Read the model definition and answer for the solid it produces. Units are mm, in the model's axes. Face numbers are marked on the shaded views. Give positions to 0.01 mm unless a question says otherwise; leave off trailing zeros. Order: outer loops, then holes, each group sorted by start corner. A loop starts at its lowest first (then second) coordinate and runs counter-clockwise, first axis right, second up.
Item 1: The mould has two halves that part along Z. Classify the marked faces 1, 2 and 3: +Z half, -Z half, draft (parallel to the pull), parting line (faces both ways), or undercut.
Item 2: A cutting plane is placed at A-A (x = 11.75). Write down the section's boundary in (y, z), plus the area to 3 significant figures.
Item 3: A cutting plane is placed at B-B (y = 10). Write down the section's boundary in (x, z), plus the area to 3 significant figures.
Item 4: A cutting plane is placed at C-C (y = 35.5). Write down the section's boundary in (x, z).
Item 5: Find the intervals of material crossed by line 1 along Y through (x, z) = (11.75, 10.4); line 2 along X through (y, z) = (17, -30); line 3 along Z through (x, y) = (14.25, 46.5), in increasing order.
Item 6: A cutting plane is placed at D-D (z = -14). Write down the section's boundary in (x, y), plus the area to 3 significant figures.
Item 7: Given pin 1 Ø3 at (y, z) = (9, -11) entering from +X; pin 2 Ø12 at (y, z) = (7.5, -20.5) entering from -X; pin 3 Ø3.5 at (x, y) = (11.75, 10) entering from -Z; pin 4 Ø8 at (y, z) = (35, -21.5) entering from -X, each flat-ended and moving along its own axis, determine where each tip first touches the part or whether it passes through.
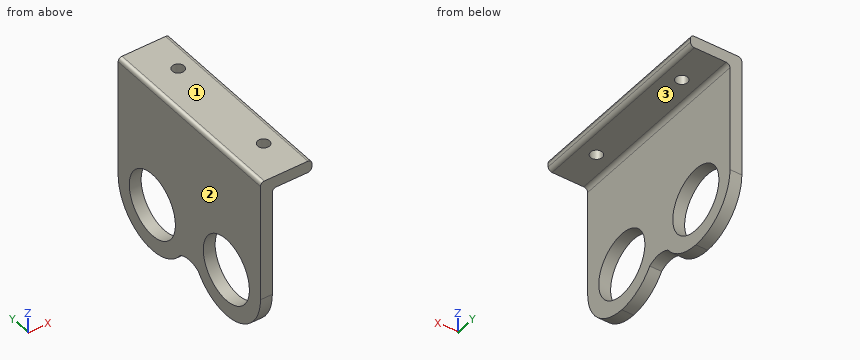
from build123d import *

# Parameters (mm, degrees)
BOSS_EXTRUDE1_DEPTH = 50
SKETCH2_R           = 1.5
CUT_EXTRUDE1_DEPTH  = 3
SKETCH3_R           = 8.1
CUT_EXTRUDE2_DEPTH  = 3


with BuildPart() as part:
    # Sketch1 → Boss-Extrude1 (new body)
    with BuildSketch(Plane(origin=(0, 0, 0), x_dir=(1, 0, 0), z_dir=(0, 1, 0))):
        with BuildLine():
            Line((3.75, 31.3125), (6.75, 31.3125))
            Line((6.75, 31.3125), (6.75, -7.6875))
            ThreePointArc((6.75, -7.6875), (7.042893219, -8.394606781), (7.75, -8.6875))
            Line((7.75, -8.6875), (15.75, -8.6875))
            ThreePointArc((15.75, -8.6875), (16.457106781, -8.980393219), (16.75, -9.6875))
            Line((16.75, -9.6875), (16.75, -10.6875))
            ThreePointArc((16.75, -10.6875), (16.457106781, -11.394606781), (15.75, -11.6875))
            Line((15.75, -11.6875), (4.75, -11.6875))
            ThreePointArc((4.75, -11.6875), (4.042893219, -11.394606781), (3.75, -10.6875))
            Line((3.75, -10.6875), (3.75, 31.3125))
        make_face()
    extrude(amount=BOSS_EXTRUDE1_DEPTH)

    # Sketch2 → Cut-Extrude1 (cut)
    with BuildSketch(Plane.XY.offset(11.6875)):
        with Locations((11.75, 40)):
            Circle(SKETCH2_R)
        with Locations((11.75, 10)):
            Circle(SKETCH2_R)
    extrude(amount=-CUT_EXTRUDE1_DEPTH, mode=Mode.SUBTRACT)

    # Sketch3 → Cut-Extrude2 (cut)
    with BuildSketch(Plane.ZY.offset(-3.75)):
        with BuildLine():
            Line((-31.3125, 0), (-19.3125, 0))
            ThreePointArc((-19.3125, 0), (-27.797781374, 3.514718626), (-31.3125, 12))
            Line((-31.3125, 12), (-31.3125, 0))
        make_face()
        with BuildLine():
            Line((-31.3125, 38), (-31.3125, 12))
            ThreePointArc((-31.3125, 12), (-29.968194023, 17.518712249), (-26.236469186, 21.800951521))
            ThreePointArc((-26.236469186, 21.800951521), (-25.3125, 25), (-26.236469186, 28.199048479))
            ThreePointArc((-26.236469186, 28.199048479), (-29.968194023, 32.481287751), (-31.3125, 38))
        make_face()
        with BuildLine():
            Line((-31.3125, 50), (-31.3125, 38))
            ThreePointArc((-31.3125, 38), (-27.797781374, 46.485281374), (-19.3125, 50))
            Line((-19.3125, 50), (-31.3125, 50))
        make_face()
        with Locations((-19.3125, 12)):
            Circle(SKETCH3_R)
        with Locations((-19.3125, 38)):
            Circle(SKETCH3_R)
    extrude(amount=-CUT_EXTRUDE2_DEPTH, mode=Mode.SUBTRACT)


solid = part.part
Response values:
1. face 1: +Z half
1. face 2: draft
1. face 3: -Z half
2. outline: (0, 8.69) - (8.5, 8.69) - (8.5, 11.69) - (0, 11.69) - close; (11.5, 8.69) - (38.5, 8.69) - (38.5, 11.69) - (11.5, 11.69) - close; (41.5, 8.69) - (50, 8.69) - (50, 11.69) - (41.5, 11.69) - close
2. area: 132 mm2
3. outline: (3.75, -31.14) - (6.75, -31.14) - (6.75, -27.16) - (3.75, -27.16) - close; (3.75, -11.46) - (6.75, -11.46) - (6.75, 7.69) arc R1 cw to (7.75, 8.69) - (10.25, 8.69) - (10.25, 11.69) - (4.75, 11.69) arc R1 ccw to (3.75, 10.69) - close; (13.25, 8.69) - (15.75, 8.69) arc R1 ccw to (16.75, 9.69) - (16.75, 10.69) arc R1 ccw to (15.75, 11.69) - (13.25, 11.69) - close
3. area: 102 mm2
4. outline: (3.75, -31.05) - (6.75, -31.05) - (6.75, -27.02) - (3.75, -27.02) - close; (3.75, -11.61) - (6.75, -11.61) - (6.75, 7.69) arc R1 cw to (7.75, 8.69) - (15.75, 8.69) arc R1 ccw to (16.75, 9.69) - (16.75, 10.69) arc R1 ccw to (15.75, 11.69) - (4.75, 11.69) arc R1 ccw to (3.75, 10.69) - close
5. line 1: y = 0 to 8.5, 11.5 to 38.5, 41.5 to 50
5. line 2: x = 3.75 to 6.75
5. line 3: z = 8.69 to 11.69
6. outline: (3.75, 0) - (6.75, 0) - (6.75, 5.89) - (3.75, 5.89) - close; (3.75, 18.11) - (6.75, 18.11) - (6.75, 31.89) - (3.75, 31.89) - close; (3.75, 44.11) - (6.75, 44.11) - (6.75, 50) - (3.75, 50) - close
6. area: 76.6 mm2
7. pin 1: stops at x = 6.75
7. pin 2: stops at x = 3.75
7. pin 3: stops at z = 8.69
7. pin 4: passes through
